Job drawing, mm, ordinate dimensions from the low corner. One solid piece. Give positions to 0.01 mm unless a question says otherwise; leave off trailing zeros. Order: outer loops, then holes, each group sorted by start corner. A loop starts at its lowest first (then second) coordinate and runs counter-clockwise, first axis right, second up. Notation, with made-up numbers: (55, 55) - (111, 55) arc R10 cw to (111, 59) - close; hole circle Ø5 at (58.5, 57). An arc over 180 degrees is marked (long way). Write each question's results on one line, items separated by ' | '. Start each with the question number.
1) Drop a flat-ended pin along its axis: pin 1 Ø3 at (x, z) = (29.8, 5.8) entering from +Y. Give the stop position or say it passes through.
2) Cut at B-B on z = 5.8. List the corners of the cut face in (x, y), plus the area to 3 significant figures.
3) Cut at A-A on x = 5.8. List the corners of the cut face in (y, z), plus the area to 3 significant figures.
4) Cut at C-C on y = 0.75. List the corners of the cut face in (x, z), plus the area to 3 significant figures.
5) Drill centre lines: line 1 along X through (y, z) = (0.9, 5.8); line 2 along Z through (x, y) = (17.8, 1.5); line 3 along X through (y, z) = (1.4, 5.25). Where is each one in solid material? Low to high. Write a range as from..to.
6) Cut at D-D on x = 41.5. List the corners of the cut face in (y, z), plus the area to 3 significant figures.
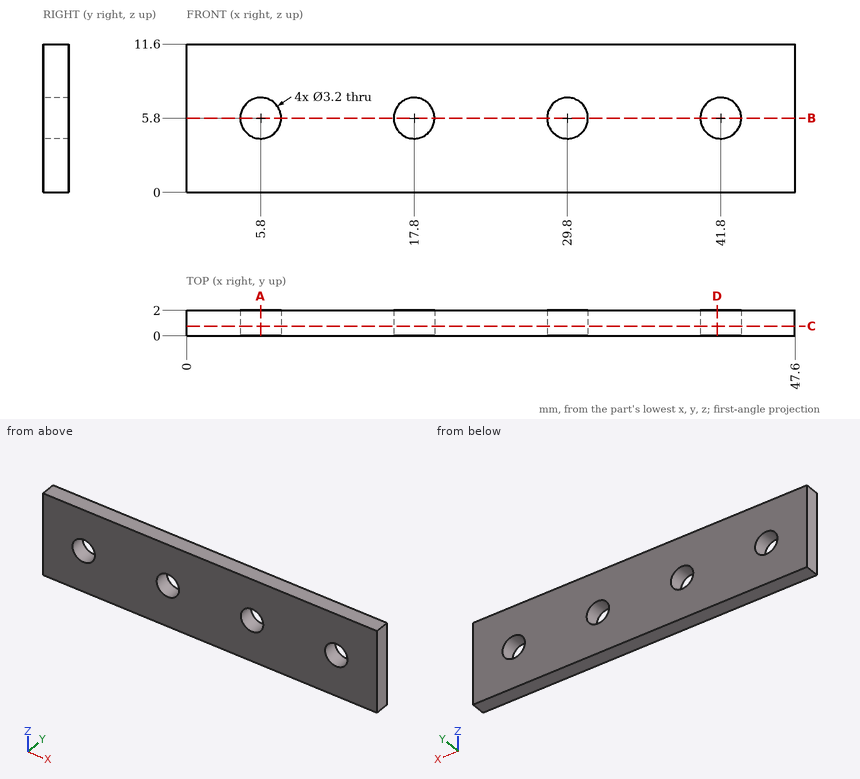
Results:
1) pin 1: through
2) outline: (0, 0) - (4.2, 0) - (4.2, 2) - (0, 2) - close; (7.4, 0) - (16.2, 0) - (16.2, 2) - (7.4, 2) - close; (19.4, 0) - (28.2, 0) - (28.2, 2) - (19.4, 2) - close; (31.4, 0) - (40.2, 0) - (40.2, 2) - (31.4, 2) - close; (43.4, 0) - (47.6, 0) - (47.6, 2) - (43.4, 2) - close | area: 69.6 mm^2
3) outline: (0, 0) - (2, 0) - (2, 4.2) - (0, 4.2) - close; (0, 7.4) - (2, 7.4) - (2, 11.6) - (0, 11.6) - close | area: 16.8 mm^2
4) outline: (0, 0) - (47.6, 0) - (47.6, 11.6) - (0, 11.6) - close; hole circle Ø3.2 at (5.8, 5.8); hole circle Ø3.2 at (17.8, 5.8); hole circle Ø3.2 at (29.8, 5.8); hole circle Ø3.2 at (41.8, 5.8) | area: 520 mm^2
5) line 1: 0..4.2, 7.4..16.2, 19.4..28.2, 31.4..40.2, 43.4..47.6 | line 2: 0..4.2, 7.4..11.6 | line 3: 0..4.3, 7.3..16.3, 19.3..28.3, 31.3..40.3, 43.3..47.6
6) outline: (0, 0) - (2, 0) - (2, 4.23) - (0, 4.23) - close; (0, 7.37) - (2, 7.37) - (2, 11.6) - (0, 11.6) - close | area: 16.9 mm^2
